Autodesk Inventor part; units mm, degrees
ref_plane "YZ Plane" through (0, 0, 0) normal (1, 0, 0) x (0, 1, 0)
ref_plane "XZ Plane" through (0, 0, 0) normal (0, 1, 0) x (-1, 0, 0)
ref_plane "XY Plane" through (0, 0, 0) normal (0, 0, 1) x (1, 0, 0)
sketch "Sketch1" plane through (0, 0, 0) normal (0, 0, 1) x (1, 0, 0)
  line L0 (-12.7, -25.4) -> (12.7, -25.4)
  line L1 (12.7, -25.4) -> (12.7, 25.4)
  line L2 (12.7, 25.4) -> (-12.7, 25.4)
  line L3 (-12.7, 25.4) -> (-12.7, -25.4)
  line L4 (-12.7, -25.4) -> (12.7, 25.4) construction
  line L5 (12.7, -25.4) -> (-12.7, 25.4) construction
  line L6 (-11.1125, 23.8125) -> (11.1125, 23.8125)
  line L7 (11.1125, 23.8125) -> (11.1125, -23.8125)
  line L8 (11.1125, -23.8125) -> (-11.1125, -23.8125)
  line L9 (-11.1125, -23.8125) -> (-11.1125, 23.8125)
  point P0 (0, 0)
  dimension "width" = 25.4
  dimension "height" = 50.8
  dimension "thickness" = 1.5875
extrude "Extrusion1" add sketch "Sketch1" along normal mid plane 387.35
sketch "Sketch2" plane through (12.7, -25.4, 193.675) normal (1, 0, 0) x (0, 0, -1)
  line L0 (387.35, 50.8) -> (387.35, 0) construction
  line L1 (387.35, 0) -> (0, 0) construction
  line L2 (0, 0) -> (0, 50.8) construction
  line L3 (0, 50.8) -> (387.35, 50.8) construction
  line L4 (387.35, 0) -> (0, 0) construction
  line L5 (0, 0) -> (0, 50.8) construction
  line L6 (0, 50.8) -> (387.35, 50.8) construction
  line L7 (387.35, 50.8) -> (387.35, 0)
  point P0 (193.675, 25.4)
  point P1 (12.7, 38.1)
  point P2 (12.7, 25.4)
  point P3 (0, 25.4)
  point P4 (12.7, 12.7)
  dimension "d5" = 12.7
  dimension "d6" = 12.7
  dimension "d7" = 12.7
hole "Hole1" at (12.7, 12.7, 180.975) at (12.7, 0, 180.975) at (12.7, -12.7, 180.975) direction (-1, 0, 0) diameter 5.1054 end through all
mirror "Mirror1" about plane through (0, 0, 0) normal (0, 0, 1) of "Hole1"
sketch "Sketch3" plane through (12.7, -25.4, 193.675) normal (1, 0, 0) x (0, 0, -1)
  circle A0 centre (374.65, 12.7) radius 2.5527 construction
  circle A1 centre (374.65, 38.1) radius 2.5527 construction
  circle A2 centre (374.65, 25.4) radius 2.5527 construction
  circle A3 centre (12.7, 25.4) radius 2.5527 construction
  circle A4 centre (12.7, 38.1) radius 2.5527 construction
  circle A5 centre (12.7, 12.7) radius 2.5527 construction
  line L0 (387.35, 50.8) -> (387.35, 0) construction
  line L1 (387.35, 0) -> (0, 0) construction
  line L2 (0, 0) -> (0, 50.8) construction
  line L3 (0, 50.8) -> (387.35, 50.8) construction
  point P0 (193.675, 25.4)
  point P1 (323.85, 25.4)
  point P2 (298.45, 25.4)
  dimension "d15" = 50.8
  dimension "d16" = 25.4
hole "Hole2" at (12.7, 0, -130.175) at (12.7, 0, -104.775) direction (-1, 0, 0) diameter 5.1054 end through all
sketch "Sketch4" plane through (12.7, -25.4, 193.675) normal (1, 0, 0) x (0, 0, -1)
  line L0 (165.1, 38.1) -> (139.7, 38.1) construction
  line L1 (165.1, 40.6527) -> (139.7, 40.6527)
  line L2 (139.7, 35.5473) -> (165.1, 35.5473)
  arc A0 (165.1, 35.5473) -> (165.1, 40.6527) centre (165.1, 38.1) ccw
  arc A1 (139.7, 40.6527) -> (139.7, 35.5473) centre (139.7, 38.1) ccw
  line L3 (165.1, 12.7) -> (139.7, 12.7) construction
  line L4 (165.1, 15.2527) -> (139.7, 15.2527)
  line L5 (139.7, 10.1473) -> (165.1, 10.1473)
  arc A2 (165.1, 10.1473) -> (165.1, 15.2527) centre (165.1, 12.7) ccw
  arc A3 (139.7, 15.2527) -> (139.7, 10.1473) centre (139.7, 12.7) ccw
  line L6 (152.4, 38.1) -> (152.4, 12.7) construction
  line L7 (0, 0) -> (0, 50.8) construction
  line L8 (101.6, 38.1) -> (76.2, 38.1) construction
  line L9 (101.6, 40.6527) -> (76.2, 40.6527)
  line L10 (76.2, 35.5473) -> (101.6, 35.5473)
  arc A4 (101.6, 35.5473) -> (101.6, 40.6527) centre (101.6, 38.1) ccw
  arc A5 (76.2, 40.6527) -> (76.2, 35.5473) centre (76.2, 38.1) ccw
  line L11 (101.6, 12.7) -> (76.2, 12.7) construction
  line L12 (101.6, 15.2527) -> (76.2, 15.2527)
  line L13 (76.2, 10.1473) -> (101.6, 10.1473)
  arc A6 (101.6, 10.1473) -> (101.6, 15.2527) centre (101.6, 12.7) ccw
  arc A7 (76.2, 15.2527) -> (76.2, 10.1473) centre (76.2, 12.7) ccw
  line L14 (88.9, 38.1) -> (88.9, 12.7) construction
  point P0 (193.675, 25.4)
  point P1 (152.4, 25.4)
  point P2 (88.9, 25.4)
  dimension "d25" = 5.1054
  dimension "d26" = 25.4
  dimension "d27" = 25.4
  dimension "d28" = 152.4
  dimension "d29" = 5.1054
  dimension "d30" = 25.4
  dimension "d31" = 25.4
  dimension "d32" = 63.5
extrude "Extrusion2" cut sketch "Sketch4" against normal through all
sketch "Sketch5" plane through (12.7, -25.4, 193.675) normal (1, 0, 0) x (0, 0, -1)
  line L0 (212.1027, 44.45) -> (212.1027, 6.35) construction
  line L1 (387.35, 50.8) -> (387.35, 0) construction
  arc A0 (165.1, 35.5473) -> (165.1, 40.6527) centre (165.1, 38.1) ccw construction
  point P0 (193.675, 25.4)
  point P1 (212.1027, 25.4)
  point P2 (387.35, 25.4)
  point P3 (167.6527, 38.1)
  dimension "d35" = 38.1
  dimension "d36" = 44.45
hole "Hole3" at (12.7, 19.05, -18.4277) at (12.7, -19.05, -18.4277) direction (-1, 0, 0) diameter 5.1054 end through all
properties part number "CL7-001" material "Aluminum 6061"
Input: part model. Units: mm. Frame: model coordinates. A direction names the side the tool comes from. Coordinates: 2 decimals unless noted, no trailing zeros. Loops run counter-clockwise (first coordinate to the right, second up) from the corner with the lowest first, then second, coordinate; pieces in that order, holes last. Notation, with made-up numbers: (17.5, 38.25) - (41.5, 38.25) arc R14 ccw to (41.5, 53.25) - close; hole circle Ø6 at (44.5, 17.5). An arc over 180 degrees is marked (long way). Answer in a Markdown table with one row per item. Add a question column.
Item 1: Mould query, pull axis Y, two halves, no side actions, for faces 3 (the flat face through (11.112, 0, -3)), 4 (the flat face through (0, -25.4, -3)), 5 (the flat face through (-12.7, 0, -3)), 6 (the flat face through (-11.112, 0, -3)). Classes: released by +Y, released by -Y, zero draft, split by the parting line, or undercut.
Item 2: Access query for faces 1 (the flat face through (12.7, 0, -3)), 2 (the flat face through (0, -23.812, -3)). Directions: +Z, -Z, +X, -X, +Y, -Y. A direction counts if a zero-diameter tool reaches every point of the face in a straight line with its end or side. Return the directions, or none.
Item 3: Section query B-B on z = -170. Return the cut outline in (x, y).
Item 4: Section query A-A on y = 6.5. Return the cut outline in (x, z) (1 decimal), then the cut area to 3 significant figures.
Item 5: Line query: line 1 along Z through (x, y) = (12.05, 12.7) (3 decimals); line 2 along Z through (x, y) = (12.1, 0) (3 decimals); line 3 along Y through (x, z) = (-6.5, -79). Output: solid intervals per line, ascending. Write a range as [from, to].
Recorded:
| question | item | result |
|---|---|---|
| 1 | face 3 | undercut |
| 1 | face 4 | released by -Y |
| 1 | face 5 | zero draft |
| 1 | face 6 | undercut |
| 2 | face 1 | +Z, -Z, +X, +Y, -Y |
| 2 | face 2 | +Z, -Z |
| 3 | outline | (-12.7, -25.4) - (12.7, -25.4) - (12.7, 25.4) - (-12.7, 25.4) - close; hole (-11.11, -23.81) - (11.11, -23.81) - (11.11, 23.81) - (-11.11, 23.81) - close |
| 4 | outline | (-12.7, -193.7) - (-11.1, -193.7) - (-11.1, 193.7) - (-12.7, 193.7) - close; (11.1, -193.7) - (12.7, -193.7) - (12.7, 193.7) - (11.1, 193.7) - close |
| 4 | area | 1,230 mm^2 |
| 5 | line 1 | [-193.675, -183.528], [-178.422, 26.022], [56.528, 89.522], [120.028, 178.422], [183.528, 193.675] |
| 5 | line 2 | [-193.675, -183.528], [-178.422, -132.728], [-127.622, -107.328], [-102.222, 178.422], [183.528, 193.675] |
| 5 | line 3 | [-25.4, -23.81], [23.81, 25.4] |
